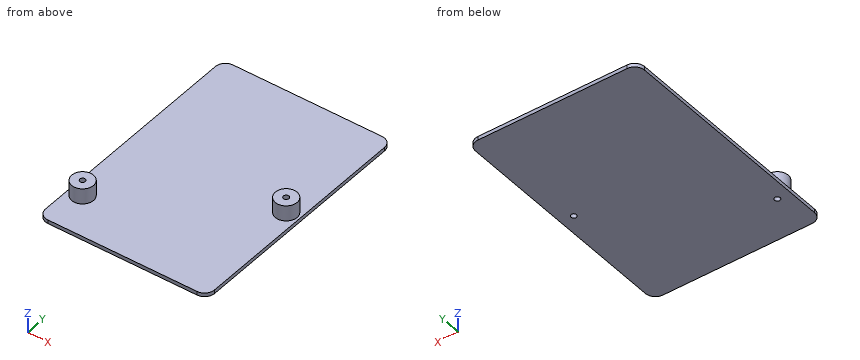
from build123d import *

# Parameters (mm, degrees)
SKETCH1_W                      = 54.4068
SKETCH1_H                      = 78.74
BOSS_EXTRUDE1_DEPTH            = 1.2
FILLET1_R                      = 3.175
CUT_EXTRUDE1_REACH             = 49.869
SKETCH2_R                      = 0.89
CUT_EXTRUDE1_DIRECTION_2_DEPTH = 48.869216325
BOSS_EXTRUDE2_START            = 5
SKETCH4_R                      = 3.5
SKETCH4_R_2                    = 0.89
BOSS_EXTRUDE2_DEPTH            = 5


with BuildPart() as part:
    # Sketch1 → Boss-Extrude1 (new body)
    with BuildSketch(Plane.XY):
        Rectangle(SKETCH1_W, SKETCH1_H)
    extrude(amount=BOSS_EXTRUDE1_DEPTH)

    # Fillet1
    fillet1_edges = [part.edges().sort_by_distance(p)[0] for p in [
        (27.2034, -39.37, 0.6),
        (-27.2034, -39.37, 0.6),
        (-27.2034, 39.37, 0.6),
        (27.2034, 39.37, 0.6),
    ]]
    fillet(fillet1_edges, radius=FILLET1_R)

    # Sketch2 → Cut-Extrude1 (cut, up to next)
    with BuildSketch(Plane.XY.offset(1.2), mode=Mode.PRIVATE) as cut_extrude1_sk1:
        with Locations(Location((-22.925, -26.04, 0), (0, 0, 180))):
            Circle(SKETCH2_R)
    cut_extrude1_tool1 = extrude(cut_extrude1_sk1.sketch, amount=-CUT_EXTRUDE1_REACH, mode=Mode.PRIVATE) & part.part
    # Sketch2 → Cut-Extrude1 (cut, up to next)
    with BuildSketch(Plane.XY.offset(1.2), mode=Mode.PRIVATE) as cut_extrude1_sk2:
        with Locations(Location((22.925, 0, 0), (0, 0, 180))):
            Circle(SKETCH2_R)
    cut_extrude1_tool2 = extrude(cut_extrude1_sk2.sketch, amount=-CUT_EXTRUDE1_REACH, mode=Mode.PRIVATE) & part.part
    add(cut_extrude1_tool1.solids().sort_by_distance((-22.925, -26.04, 1.2))[0], mode=Mode.SUBTRACT)
    add(cut_extrude1_tool2.solids().sort_by_distance((22.925, 0, 1.2))[0], mode=Mode.SUBTRACT)

    # Sketch2 → Cut-Extrude1 direction 2 (cut)
    with BuildSketch(Plane.XY.offset(1.2)):
        with Locations(Location((-22.925, -26.04, 0), (0, 0, 180))):
            Circle(SKETCH2_R)
        with Locations(Location((22.925, 0, 0), (0, 0, 180))):
            Circle(SKETCH2_R)
    extrude(amount=CUT_EXTRUDE1_DIRECTION_2_DEPTH, mode=Mode.SUBTRACT)

    # Sketch4 → Boss-Extrude2 (add)
    # profile 1 of 2: a face of its own
    with BuildSketch(Plane.XY.offset(1.2).offset(BOSS_EXTRUDE2_START)):
        with Locations(Location((-22.925, -26.04, 0), (0, 0, 180))):
            Circle(SKETCH4_R)
        with Locations(Location((-22.925, -26.04, 0), (0, 0, 180))):
            Circle(SKETCH4_R_2, mode=Mode.SUBTRACT)
    # profile 2 of 2: a face of its own
    with BuildSketch(Plane.XY.offset(1.2).offset(BOSS_EXTRUDE2_START)):
        with Locations(Location((22.925, 0, 0), (0, 0, 180))):
            Circle(SKETCH4_R)
        with Locations(Location((22.925, 0, 0), (0, 0, 180))):
            Circle(SKETCH4_R_2, mode=Mode.SUBTRACT)
    extrude(amount=-BOSS_EXTRUDE2_DEPTH)


solid = part.part
Work out the finished part from the listing and answer in its coordinate system (mm). Give positions to 0.01 mm unless a question says otherwise; leave off trailing zeros. Loops run counter-clockwise (first coordinate to the right, second up) from the corner with the lowest first, then second, coordinate; pieces in that order, holes last. Notation, with made-up numbers: (20.5, 54) - (43.5, 54) arc R19 cw to (43.5, 73) - close; hole circle Ø8 at (25.5, 3). An arc over 180 degrees is marked (long way). Answer in a Markdown table with one row per item.
(1) Section A-A (y = 0) is taken. Give the vertices of the cut face in (x, z) (3 decimals).
Results list:
| item | result |
|---|---|
| outline | (-27.203, 0) - (22.035, 0) - (22.035, 6.2) - (19.425, 6.2) - (19.425, 1.2) - (-27.203, 1.2) - close; (23.815, 0) - (27.203, 0) - (27.203, 1.2) - (26.425, 1.2) - (26.425, 6.2) - (23.815, 6.2) - close |
(2) Flat-ended cylindrical pins translate along their axes: pin 1 Ø2 at (x, z) = (-9, 4) entering from -Y; pin 2 Ø12 at (x, y) = (-17.5, -25) entering from +Z; pin 3 Ø3 at (y, z) = (-1.5, 3) entering from +X (3 decimals); pin 4 Ø12 at (x, y) = (-5, -26) entering from +Z. Find the tip coordinate at first contact, or state that the pin passes through.
Results list:
| item | result |
|---|---|
| pin 1 | passes through |
| pin 2 | stops at z = 6.2 |
| pin 3 | stops at x = 26.425 |
| pin 4 | stops at z = 1.2 |
(3) Consider L1, parallel to X at y = -26.04, z = 3 (3 decimals); L2, parallel to Z at x = -18.5, y = 3; L3, parallel to X at y = -2, z = 2.25. Determine where each line is inside the solid, lowest interval first. Write a range as [from, to].
Results list:
| item | result |
|---|---|
| L1 | x = [-26.425, -23.815], [-22.035, -19.425] |
| L2 | z = [0, 1.2] |
| L3 | x = [20.05, 25.8] |
(4) Section D-D (y = -19.5) is taken. Give the vertices of the cut face in (x, z).
Results list:
| item | result |
|---|---|
| outline | (-27.2, 0) - (27.2, 0) - (27.2, 1.2) - (-27.2, 1.2) - close |
(5) Section B-B (z = 2.5) is taken. Give the vertices of the cut face in (x, y) (3 decimals), and give its area (3 significant figures).
Results list:
| item | result |
|---|---|
| outline | circle Ø7 at (-22.925, -26.04); circle Ø7 at (22.925, 0); hole circle Ø1.78 at (-22.925, -26.04); hole circle Ø1.78 at (22.925, 0) |
| area | 72.0 mm² |
(6) Section C-C (x = 20.5) is taken. Give the vertices of the cut face in (y, z), and give its area (3 significant figures).
Results list:
| item | result |
|---|---|
| outline | (-39.37, 0) - (39.37, 0) - (39.37, 1.2) - (2.52, 1.2) - (2.52, 6.2) - (-2.52, 6.2) - (-2.52, 1.2) - (-39.37, 1.2) - close |
| area | 120 mm² |
